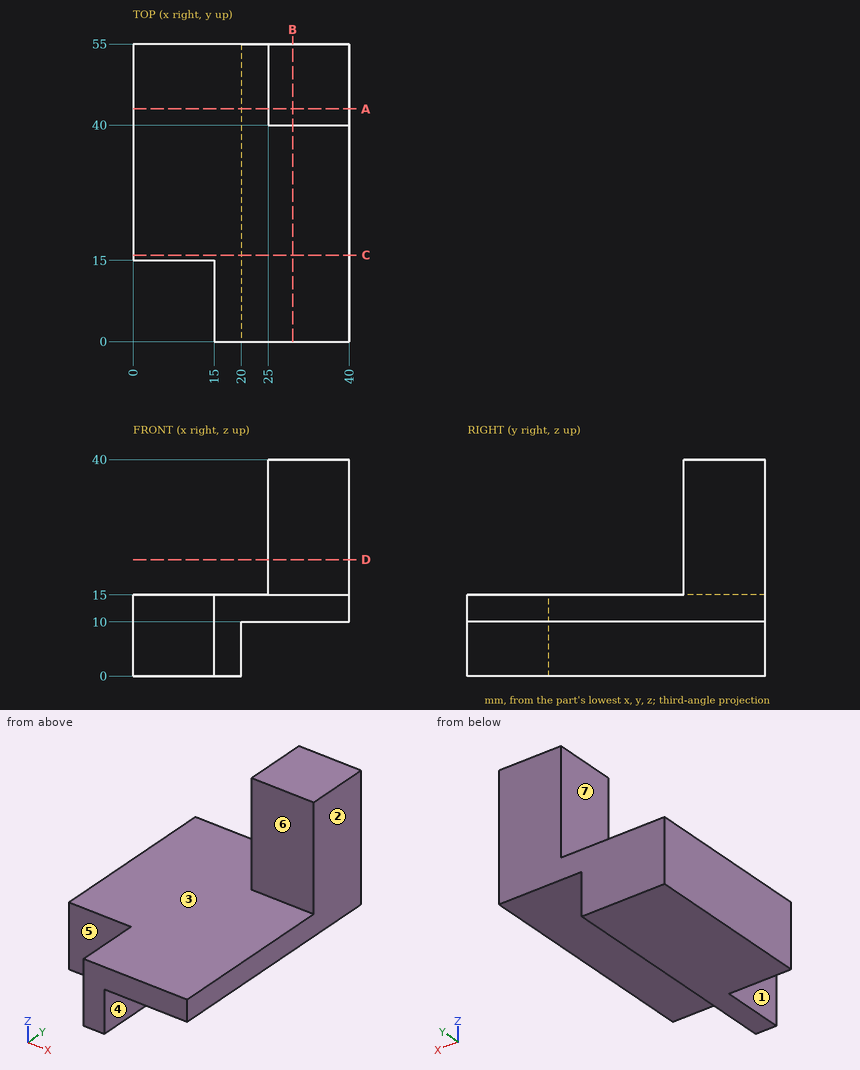
Study the drawing (mm; zero at the part's minimum x, y, z) and answer. A direction names the side the tool comes from. Coordinates: 2 decimals unless noted, no trailing zeros. Loops run counter-clockwise (first coordinate to the right, second up) from the corner with the lowest first, then second, coordinate; pieces in that order, holes last. Notation, with made-up numbers: M 38,34.5 L 83,34.5 A11 cw 83,53.5 Z; hole C 0,73 d3. An arc over 180 degrees is marked long. Answer as a JSON object with one key per item and string values. Group by question number.
Item 1: Section B-B (x = 29.5) is taken. Write down the section's boundary in (y, z).
Item 2: Section C-C (y = 16) is taken. Write down the section's boundary in (x, z).
Item 3: Determine the mould class of the marked faces 1, 2 and 3 for opening direction X: +X half, -X half, draft (parallel to the pull), parting line (faces both ways), or undercut.
Item 4: Which of the six approach directions +Z, -Z, +X, -X, +Y, -Y give full straight-line access (tool end or side, diameter ignored) to the marked faces 4, 5, 6 and 7?
Item 5: Section A-A (y = 43) is taken. Write down the section's boundary in (x, z), and give its area (3 significant figures).
Item 6: Section D-D (z = 21.5) is taken. Write down the section's boundary in (x, y).
Item 7: Consider L1, parallel to X at y = 30.5, z = 2; L2, parallel to Z at x = 14.5, y = 53.5; L3, parallel to Z at x = 25.5, y = 13. Determine where each line is inside the solid, lowest interval first.
Item 8: Each of these flat-tipped pins is pushed along its axis until it touches: P1, Ø5, axis at y = 29, z = 4.5, coming from the +X side; P2, Ø16.5, axis at y = 44.5, z = 26.5, coming from the -X side; P3, Ø6, axis at x = 34, y = 37.5, coming from the -Z side. Where does it stop, or does it pass through?
Solved:
{
 "1": {"outline": "M 0,10 L 55,10 L 55,40 L 40,40 L 40,15 L 0,15 Z"},
 "2": {"outline": "M 0,0 L 20,0 L 20,10 L 40,10 L 40,15 L 0,15 Z"},
 "3": {"face 1": "-X half", "face 2": "+X half", "face 3": "draft"},
 "4": {"face 4": "-Z, +X, +Y, -Y", "face 5": "+Z, -Z, -X, -Y", "face 6": "+Z, +X, -X, -Y", "face 7": "+Z, -X, +Y, -Y"},
 "5": {"outline": "M 0,0 L 20,0 L 20,10 L 40,10 L 40,40 L 25,40 L 25,15 L 0,15 Z", "area": "775 mm2"},
 "6": {"outline": "M 25,40 L 40,40 L 40,55 L 25,55 Z"},
 "7": {"L1": "x = 0 to 20", "L2": "z = 0 to 15", "L3": "z = 10 to 15"},
 "8": {"P1": "stops at x = 20", "P2": "stops at x = 25", "P3": "stops at z = 10"}
}
